from build123d import *

# Parameters (mm, degrees)
SKETCH1_R               = 18.5
BOSS_EXTRUDE1_DEPTH     = 45
SKETCH1_3_R             = 18.5
BOSS_EXTRUDE2_DEPTH     = 1
CUT_EXTRUDE1_REACH      = 55.648
CUT_EXTRUDE1_END_RADIUS = 21.5
SKETCH2_W               = 6
SKETCH2_H               = 6
SKETCH2_W_2             = 18.211242215
SKETCH2_H_2             = 14.156014421
SKETCH3_W               = 4
SKETCH3_H               = 2
BOSS_EXTRUDE3_DEPTH     = 8.5


with BuildPart() as part:
    # Sketch1 → Boss-Extrude1 (new body)
    with BuildSketch(Plane(origin=(0, 0, 0), x_dir=(1, 0, 0), z_dir=(0, 1, 0))):
        with BuildLine():
            ThreePointArc((19.769048133, 8.451907235), (0, 21.5), (-19.769048133, 8.451907235))
            Line((-19.769048133, 8.451907235), (-19.769048133, -8.451907235))
            ThreePointArc((-19.769048133, -8.451907235), (0, -21.5), (19.769048133, -8.451907235))
            Line((19.769048133, -8.451907235), (19.769048133, 8.451907235))
        make_face()
        with Locations(Location((0, 0, 0), (0, 0, 90))):
            Circle(SKETCH1_R, mode=Mode.SUBTRACT)
    extrude(amount=BOSS_EXTRUDE1_DEPTH)

    # Sketch1_3 → Boss-Extrude2 (add)
    with BuildSketch(Plane(origin=(0, 0, 0), x_dir=(1, 0, 0), z_dir=(0, 1, 0))):
        with Locations(Location((0, 0, 0), (0, 0, 90))):
            Circle(SKETCH1_3_R)
    extrude(amount=BOSS_EXTRUDE2_DEPTH)

    # Cut-Extrude1: up to this cylinder (the profile starts inside it)
    cut_extrude1_end = Plane(origin=(0, 11.2781055, 0), z_dir=(0, -1, 0)) * Cylinder(CUT_EXTRUDE1_END_RADIUS, 169.852211, mode=Mode.PRIVATE)
    # Sketch2 → Cut-Extrude1 (cut, up to the surface)
    with BuildSketch(Plane.XY, mode=Mode.PRIVATE) as cut_extrude1_sk1:
        with Locations((0.640621421, 4)):
            Rectangle(SKETCH2_W, SKETCH2_H)
    cut_extrude1_tool1 = extrude(cut_extrude1_sk1.sketch, amount=CUT_EXTRUDE1_REACH, mode=Mode.PRIVATE) & cut_extrude1_end
    add(cut_extrude1_tool1.solids().sort_by_distance((0.640621, 4, 0))[0], mode=Mode.SUBTRACT)
    # Sketch2 → Cut-Extrude1 (cut, up to the surface)
    with BuildSketch(Plane.XY, mode=Mode.PRIVATE) as cut_extrude1_sk2:
        with Locations((0.419944281, 18.556211079)):
            Rectangle(SKETCH2_W_2, SKETCH2_H_2)
    cut_extrude1_tool2 = extrude(cut_extrude1_sk2.sketch, amount=CUT_EXTRUDE1_REACH, mode=Mode.PRIVATE) & cut_extrude1_end
    add(cut_extrude1_tool2.solids().sort_by_distance((0.419944, 18.556211, 0))[0], mode=Mode.SUBTRACT)

    # Sketch3 → Boss-Extrude3 (add, symmetric)
    with BuildSketch(Plane.XY):
        with Locations((-21.769048133, 1)):
            Rectangle(SKETCH3_W, SKETCH3_H)
    boss_extrude3 = extrude(amount=BOSS_EXTRUDE3_DEPTH, both=True)

    # Mirror1: Boss-Extrude3 across plane
    add(boss_extrude3.mirror(Plane(origin=(0, 0, 0), x_dir=(0, 0, 1), z_dir=(1, 0, 0))))


solid = part.part
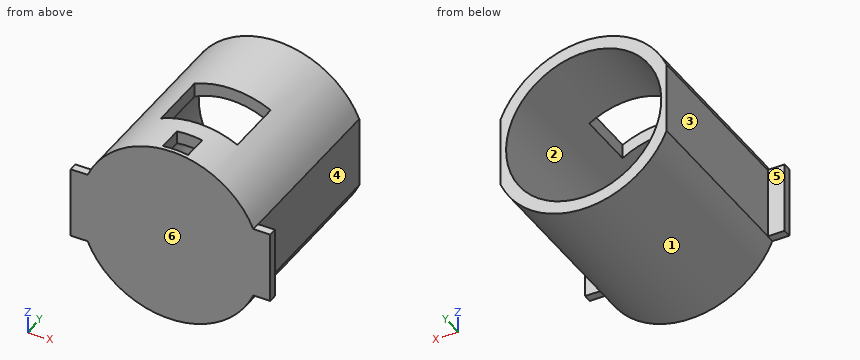
Here's how the part is built. I have some questions about the finished solid (model axes, mm). Face numbers are marked on the shaded views. A direction names the side the tool comes from. Give positions to 0.01 mm unless a question says otherwise; leave off trailing zeros. Loops run counter-clockwise (first coordinate to the right, second up) from the corner with the lowest first, then second, coordinate; pieces in that order, holes last. Notation, with made-up numbers: (13, 52.25) -> (36, 52.25) arc R24 cw to (36, 86.25) -> close; hole circle Ø6 at (13, 46). An arc over 180 degrees is marked (long way). Answer as a JSON object with one key per item and string values. Group by question number.
Item 1: I need wall thicknesses on L1, parallel to X at y = 24.5, z = 0; L2, parallel to Y at x = -6, z = 3; L3, parallel to X at y = 3.5, z = -11.5. Which ranges of each line are inside material? Lowest first, please.
Item 2: Imagine slicing it at A-A on x = 0. Write out the boundary of the cut face in (y, z).
Item 3: Imagine slicing it at B-B on z = 6. Write out the boundary of the cut face in (x, y).
Item 4: Will these pins go through, and if not, where does the flat tip stop? pin 1 (4 mm diameter, centred on x = 14, y = 32.5, fed in from -Z); pin 2 (4.5 mm diameter, centred on x = -0.5, z = 19, fed in from -Y); pin 3 (1.7 mm diameter, centred on y = 15, z = 18.5, fed in from -X); pin 4 (6 mm diameter, centred on y = 30, z = -7.5, fed in from -X).
Item 5: Imagine slicing it at C-C on y = 39. Write out the boundary of the cut face in (x, z).
Item 6: Imagine slicing it at D-D on x = 7. Write out the boundary of the cut face in (y, z), then the cut area to 3 significant figures.
Item 7: On a 3-axis mill with a long thin cutter (end or side, diameter ignored), from which of +Z, -Z, +X, -X, +Y, -Y can I reach the whole of each face in a straight line? I mean the marked faces 4, 5 and 6. Say none if no direction works.
Item 8: Thinking about a two-plate mould opening in Z: for the marked faces 1, 2 and 3, which applies, pulls with the +Z half, pulls with the -Z half, needs draft (parallel to the pull), parting line crosses it, or undercut?
Answer list:
{
 "1": {"L1": "x = -19.77 to -18.5, 18.5 to 19.77", "L2": "y = 0 to 1", "L3": "x = -18.17 to -14.49, 14.49 to 18.17"},
 "2": {"outline": "(0, -21.5) -> (45, -21.5) -> (45, -18.5) -> (1, -18.5) -> (1, 21.5) -> (0, 21.5) -> close; (7, 18.5) -> (11.48, 18.5) -> (11.48, 21.5) -> (7, 21.5) -> close; (25.63, 18.5) -> (45, 18.5) -> (45, 21.5) -> (25.63, 21.5) -> close"},
 "3": {"outline": "(-23.77, 0) -> (23.77, 0) -> (23.77, 2) -> (19.77, 2) -> (19.77, 45) -> (17.5, 45) -> (17.5, 1) -> (-17.5, 1) -> (-17.5, 45) -> (-19.77, 45) -> (-19.77, 2) -> (-23.77, 2) -> close"},
 "4": {"pin 1": "stops at z = -17.84", "pin 2": "stops at y = 0", "pin 3": "stops at x = -12.28", "pin 4": "stops at x = -19.77"},
 "5": {"outline": "(-19.77, -8.45) arc R21.5 ccw to (19.77, -8.45) -> (19.77, 8.45) arc R21.5 ccw to (-19.77, 8.45) -> close; hole circle Ø37 at (0, 0)"},
 "6": {"outline": "(0, -20.33) -> (45, -20.33) -> (45, -17.12) -> (1, -17.12) -> (1, 17.12) -> (11.48, 17.12) -> (11.48, 20.33) -> (0, 20.33) -> close; (25.63, 17.12) -> (45, 17.12) -> (45, 20.33) -> (25.63, 20.33) -> close", "area": "277 mm2"},
 "7": {"face 4": "+Z, -Z, +X, +Y", "face 5": "+Z, -Z, -X, +Y", "face 6": "+Z, -Z, +X, -X, -Y"},
 "8": {"face 1": "pulls with the -Z half", "face 2": "undercut", "face 3": "needs draft"}
}
